Geometry: see drawing. Coordinates: mm, zero at the bounding-box minimum. A direction names the side the tool comes from. Give positions to 0.01 mm unless a question says otherwise; leave off trailing zeros. Write each loop counter-clockwise with the first axis right and the second up, starting at its lowest first coordinate (ties: lowest second). Pieces come first, ordered by that corner, then holes. Notation, with made-up numbers: (5, 67) -> (29, 67) arc R20 ccw to (29, 88) -> close; hole circle Ø6 at (69.25, 39). An arc over 180 degrees is marked (long way). Answer as a JSON object with one key per item and string values. Group by question number.
Item 1: Section query B-B on z = 1033.5. Return the cut outline in (x, y), plus the area to 3 significant figures.
Item 2: First-contact query: pin 1 Ø15 at (x, z) = (1008, 1057) entering from -Y; pin 2 Ø3 at (x, y) = (891.5, 223.5) entering from -Z; pin 3 Ø9.5 at (y, z) = (547.5, 18.5) entering from +X. Flat tips, straight axial feed; report the tip coordinate or a pass-through.
Item 3: Ray query, probe 1 along Z at (x, y) = (288, 109.5); probe 2 along X at (y, z) = (184.5, 1616). Return the intervals inside material, ascending. Write a range as from..to.
Item 4: Section query C-C on y = 50.5. Return the cut outline in (x, z).
Item 5: Access query for the marked faces 1 and 2. Directions: +Z, -Z, +X, -X, +Y, -Y. A direction counts if a zero-diameter tool reaches every point of the face in a straight line with its end or side. Return the directions, or none.
Item 6: Section query D-D on y = 380.5. Return the cut outline in (x, z), plus the area to 3 significant figures.
Item 7: Section query A-A on x = 198.5. Return the cut outline in (y, z), plus the area to 3 significant figures.
Item 8: Pull-direction query (Z, two-part tool) for the marked faces 3, 4 and 5; classes: pulls with the +Z half, pulls with the -Z half, needs draft (parallel to the pull), parting line crosses it, or undercut.
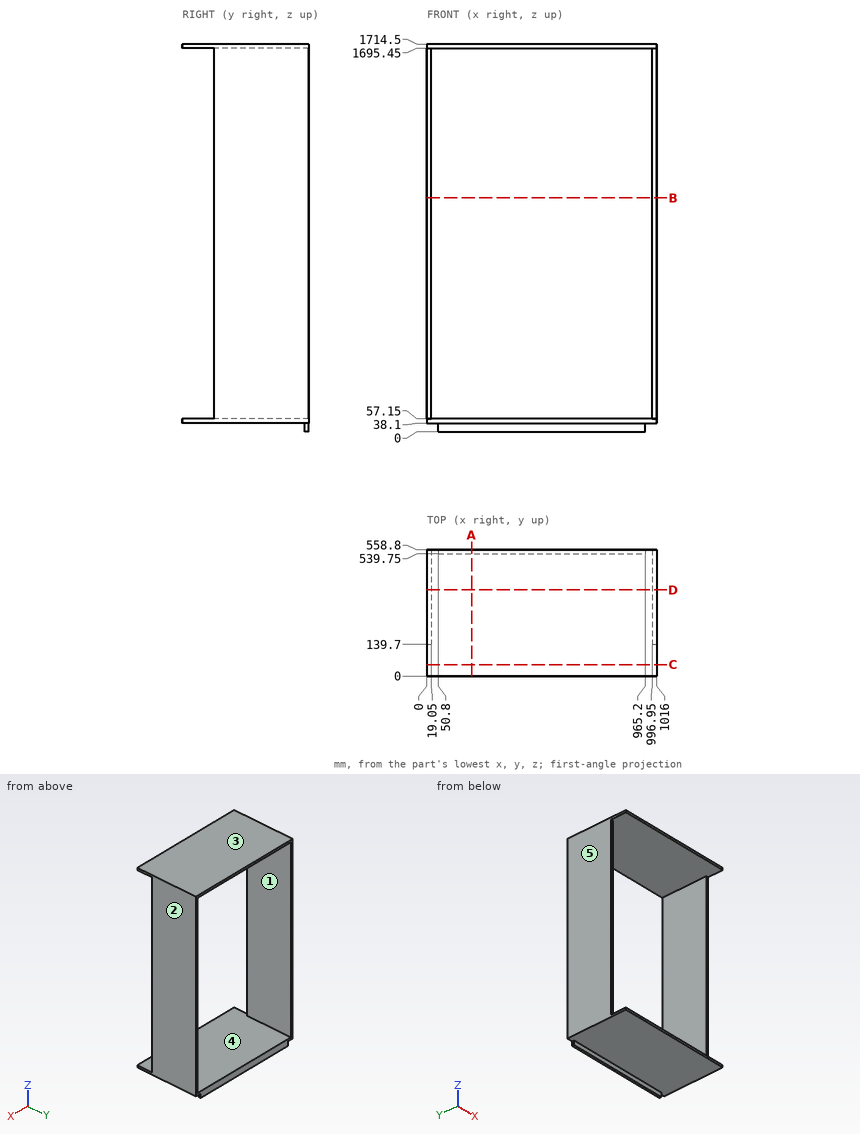
Worked answers:
{
 "1": {"outline": "(0, 139.7) -> (19.05, 139.7) -> (19.05, 558.8) -> (0, 558.8) -> close; (996.95, 139.7) -> (1016, 139.7) -> (1016, 558.8) -> (996.95, 558.8) -> close", "area": "16,000 mm^2"},
 "2": {"pin 1": "y = 139.7", "pin 2": "z = 38.1", "pin 3": "x = 965.2"},
 "3": {"probe 1": "38.1..57.15, 1695.45..1714.5", "probe 2": "0..19.05, 996.95..1016"},
 "4": {"outline": "(0, 38.1) -> (1016, 38.1) -> (1016, 57.15) -> (0, 57.15) -> close; (0, 1695.45) -> (1016, 1695.45) -> (1016, 1714.5) -> (0, 1714.5) -> close"},
 "5": {"face 1": "+Y, -Y", "face 2": "+Z, -Z, +X, +Y, -Y"},
 "6": {"outline": "(0, 38.1) -> (1016, 38.1) -> (1016, 1714.5) -> (0, 1714.5) -> close; hole (19.05, 57.15) -> (996.95, 57.15) -> (996.95, 1695.45) -> (19.05, 1695.45) -> close", "area": "101,000 mm^2"},
 "7": {"outline": "(0, 38.1) -> (539.75, 38.1) -> (539.75, 0) -> (558.8, 0) -> (558.8, 57.15) -> (0, 57.15) -> close; (0, 1695.45) -> (558.8, 1695.45) -> (558.8, 1714.5) -> (0, 1714.5) -> close", "area": "22,000 mm^2"},
 "8": {"face 3": "pulls with the +Z half", "face 4": "undercut", "face 5": "needs draft"}
}
